Could you check a few things on this model? Use its own coordinates, in mm. Coordinates: 2 decimals unless noted, no trailing zeros. Loops run counter-clockwise (first coordinate to the right, second up) from the corner with the lowest first, then second, coordinate; pieces in that order, holes last. Notation, with made-up numbers: (37, -21) - (68, -21) arc R18 ccw to (68, -5) - close; hole circle Ø7 at (84, -26). An arc over 180 degrees is marked (long way). One line per item, written item: value. Start each with the question number.
(1) If I drill on line 1 along X through (y, z) = (1.95, -112); line 2 along X through (y, z) = (1.6, -29); line 3 along X through (y, z) = (2.25, -136), over which ranges is the centre line in solid material (lowest first)? Write a range as from..to.
(2) If we section it at A-A on z = -4: Write out the boundary of the cut face in (x, y).
(3) If we section it at B-B on y = 4: Count the separate pieces of the cut face and the enclosed holes in it, then the cut area to 3 significant figures.
```python
from build123d import *

# Parameters (mm, degrees)
SKETCH1_R           = 1.6
SKETCH1_W           = 5.099999999
SKETCH1_H           = 15
SKETCH1_W_2         = 5.099999998
SKETCH1_W_3         = 5.1
BOSS_EXTRUDE1_DEPTH = 5


with BuildPart() as part:
    # Sketch1 → Boss-Extrude1 (new body)
    with BuildSketch(Plane(origin=(0, 0, 0), x_dir=(1, 0, 0), z_dir=(0, 1, 0))):
        with BuildLine():
            Line((-42.697719413, 225.280869355), (192.302280587, 225.280869355))
            ThreePointArc((192.302280587, 225.280869355), (199.373348399, 222.351937167), (202.302280587, 215.280869355))
            Line((202.302280587, 215.280869355), (202.302280587, -24.719130645))
            ThreePointArc((202.302280587, -24.719130645), (199.373348399, -31.790198457), (192.302280587, -34.719130645))
            Line((192.302280587, -34.719130645), (94.802280587, -34.719130645))
            ThreePointArc((94.802280587, -34.719130645), (87.731212775, -31.790198457), (84.802280587, -24.719130645))
            Line((84.802280587, -24.719130645), (84.802280587, 60.280869355))
            ThreePointArc((84.802280587, 60.280869355), (83.337814493, 63.816403261), (79.802280587, 65.280869355))
            Line((79.802280587, 65.280869355), (69.802280587, 65.280869355))
            ThreePointArc((69.802280587, 65.280869355), (66.266746681, 63.816403261), (64.802280587, 60.280869355))
            Line((64.802280587, 60.280869355), (64.802280587, -24.719130645))
            ThreePointArc((64.802280587, -24.719130645), (61.873348399, -31.790198457), (54.802280587, -34.719130645))
            Line((54.802280587, -34.719130645), (-42.697719413, -34.719130645))
            ThreePointArc((-42.697719413, -34.719130645), (-49.768787225, -31.790198457), (-52.697719413, -24.719130645))
            Line((-52.697719413, -24.719130645), (-52.697719413, 215.280869355))
            ThreePointArc((-52.697719413, 215.280869355), (-49.768787225, 222.351937167), (-42.697719413, 225.280869355))
        make_face()
        with Locations(Location((192.302280587, 135.280869355, 0), (0, 0, 270))):
            Circle(SKETCH1_R, mode=Mode.SUBTRACT)
        with Locations(Location((-42.697719413, 135.280869355, 0), (0, 0, 270))):
            Circle(SKETCH1_R, mode=Mode.SUBTRACT)
        with Locations((192.302280588, 157.780869355)):
            Rectangle(SKETCH1_W, SKETCH1_H, mode=Mode.SUBTRACT)
        with Locations((192.302280587, 112.780869355)):
            Rectangle(SKETCH1_W_2, SKETCH1_H, mode=Mode.SUBTRACT)
        with Locations((-42.697719413, 157.780869355)):
            Rectangle(SKETCH1_W_3, SKETCH1_H, mode=Mode.SUBTRACT)
        with Locations((-42.697719413, 112.780869355)):
            Rectangle(SKETCH1_W_3, SKETCH1_H, mode=Mode.SUBTRACT)
    extrude(amount=BOSS_EXTRUDE1_DEPTH)


solid = part.part
```
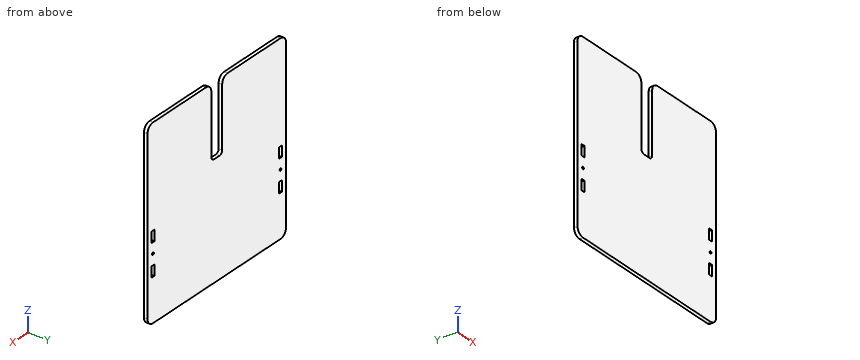
Values:
1. line 1: x = -52.7..-45.25, -40.15..189.75, 194.85..202.3
1. line 2: x = -52.7..64.8, 84.8..202.3
1. line 3: x = -52.7..-44.13, -41.27..190.87, 193.73..202.3
2. outline: (-52.7, 0) - (64.8, 0) - (64.8, 5) - (-52.7, 5) - close; (84.8, 0) - (202.3, 0) - (202.3, 5) - (84.8, 5) - close
3. separate pieces: 1
3. enclosed holes: 6
3. area: 63,900 mm2
